Geometry check sheet. Reference: the model listing, model coordinates, mm. Face numbers are marked on the shaded views. A direction names the side the tool comes from. Coordinates: 2 decimals unless noted, no trailing zeros. Order: outer loops, then holes, each group sorted by start corner. A loop starts at its lowest first (then second) coordinate and runs counter-clockwise, first axis right, second up. Notation, with made-up numbers: M 25.5,5 L 61.5,5 A37 cw 61.5,44 Z; hole C 11,-30.5 d3. An arc over 180 degrees is marked long. Use CSV: the item, a comma, the result in double quotes. Start each with the question number.
```python
from build123d import *

# Parameters (mm, degrees)
FURO_ROSCADO_DE_1_4_18_NPSM1_REACH  = 69.594
FURO_ROSCADO_DE_1_4_18_NPSM1_BORE_R = 5.9436
FURO_ROSCADO_DE_1_4_18_NPSM2_REACH  = 82.554
FURO_ROSCADO_DE_1_4_18_NPSM2_BORE_R = 5.9436
ESBO_O4_R                           = 10
CORTE_EXTRUS_O1_DEPTH               = 2
ESBO_O6_R                           = 10
CORTE_EXTRUS_O2_DEPTH               = 2
CORTE_EXTRUS_O3_DEPTH               = 79.42193586


with BuildPart() as part:
    # Esboço1 → Revolução1 (revolve)
    with BuildSketch(Plane.XY, mode=Mode.PRIVATE) as revolu_o1_sk:
        Polygon((9, 32), (25, 32), (25, -38), (0, -38), (0, -34), (9, -34), align=None)
    revolve(revolu_o1_sk.sketch.rotate(Axis((0, 0, 0), (0, 1, 0)), 90), axis=Axis((0, 0, 0), (0, 1, 0)))

    # Furo roscado de 1/4-18 NPSM1 bore (on position points) → Furo roscado de 1/4-18 NPSM1 (cut, up to next)
    with BuildSketch(Plane(origin=(-25, 0, 0), x_dir=(0, 0, -1), z_dir=(-1, 0, 0)), mode=Mode.PRIVATE) as furo_roscado_de_1_4_18_npsm1_sk1:
        Circle(FURO_ROSCADO_DE_1_4_18_NPSM1_BORE_R)
    furo_roscado_de_1_4_18_npsm1_tool1 = extrude(furo_roscado_de_1_4_18_npsm1_sk1.sketch, amount=-FURO_ROSCADO_DE_1_4_18_NPSM1_REACH, mode=Mode.PRIVATE) & part.part
    add(furo_roscado_de_1_4_18_npsm1_tool1.solids().sort_by_distance((-25, 0, 0))[0], mode=Mode.SUBTRACT)

    # Furo roscado de 1/4-18 NPSM2 bore (on position points) → Furo roscado de 1/4-18 NPSM2 (cut, up to next)
    with BuildSketch(Plane(origin=(25, 20, 0), x_dir=(0, 0, 1), z_dir=(1, 0, 0)), mode=Mode.PRIVATE) as furo_roscado_de_1_4_18_npsm2_sk1:
        Circle(FURO_ROSCADO_DE_1_4_18_NPSM2_BORE_R)
    furo_roscado_de_1_4_18_npsm2_tool1 = extrude(furo_roscado_de_1_4_18_npsm2_sk1.sketch, amount=-FURO_ROSCADO_DE_1_4_18_NPSM2_REACH, mode=Mode.PRIVATE) & part.part
    # Furo roscado de 1/4-18 NPSM2 bore (on position points) → Furo roscado de 1/4-18 NPSM2 (cut, up to next)
    with BuildSketch(Plane(origin=(25, 20, 0), x_dir=(0, 0, 1), z_dir=(1, 0, 0)), mode=Mode.PRIVATE) as furo_roscado_de_1_4_18_npsm2_sk2:
        with Locations((0, 40)):
            Circle(FURO_ROSCADO_DE_1_4_18_NPSM2_BORE_R)
    furo_roscado_de_1_4_18_npsm2_tool2 = extrude(furo_roscado_de_1_4_18_npsm2_sk2.sketch, amount=-FURO_ROSCADO_DE_1_4_18_NPSM2_REACH, mode=Mode.PRIVATE) & part.part
    add(furo_roscado_de_1_4_18_npsm2_tool1.solids().sort_by_distance((25, 20, 0))[0], mode=Mode.SUBTRACT)
    add(furo_roscado_de_1_4_18_npsm2_tool2.solids().sort_by_distance((25, -20, 0))[0], mode=Mode.SUBTRACT)

    # Esboço4 → Corte-extrusão1 (cut)
    with BuildSketch(Plane(origin=(-25, 0, 0), x_dir=(0, 0, -1), z_dir=(1, 0, 0))):
        Circle(ESBO_O4_R)
    extrude(amount=CORTE_EXTRUS_O1_DEPTH, mode=Mode.SUBTRACT)

    # Esboço6 → Corte-extrusão2 (cut)
    with BuildSketch(Plane(origin=(25, 0, 0), x_dir=(0, 0, -1), z_dir=(1, 0, 0))):
        with Locations((0, 20)):
            Circle(ESBO_O6_R)
        with Locations((0, -20)):
            Circle(ESBO_O6_R)
    extrude(amount=-CORTE_EXTRUS_O2_DEPTH, mode=Mode.SUBTRACT)

    # Esboço7 → Corte-extrusão3 (cut, through all)
    with BuildSketch(Plane(origin=(0, 32, 0), x_dir=(1, 0, 0), z_dir=(0, 1, 0))):
        with BuildLine():
            Line((-20.712315177, 14), (20.712315177, 14))
            ThreePointArc((20.712315177, 14), (0, 25), (-20.712315177, 14))
        make_face()
        with BuildLine():
            Line((-20.712315177, -14), (20.712315177, -14))
            ThreePointArc((20.712315177, -14), (0, -25), (-20.712315177, -14))
        make_face()
    extrude(amount=-CORTE_EXTRUS_O3_DEPTH, mode=Mode.SUBTRACT)


solid = part.part
```
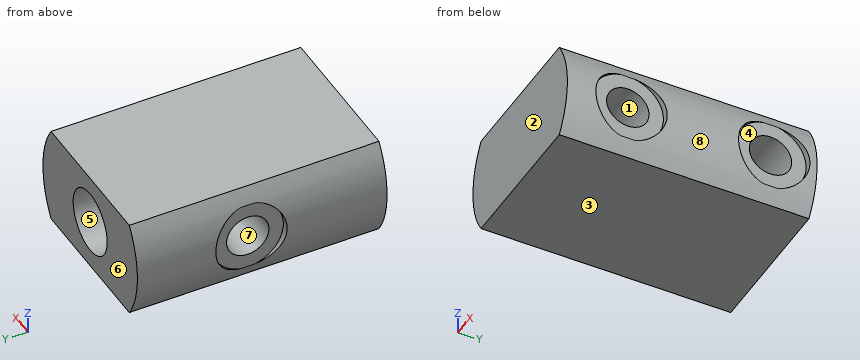
1) Gauge pin test, flat ends, axial feed: P1, Ø7, axis at y = 0, z = 0, coming from the -X side; P2, Ø6, axis at y = -21.5, z = -7.5, coming from the -X side; P3, Ø12, axis at y = 10.5, z = -6.5, coming from the -X side (3 decimals). Record the tip position at first contact, or that the pin passes through.
2) Set-up check for the marked faces 4, 5, 6, 7 and 8: record each of +Z, -Z, +X, -X, +Y, -Y from which the full face is reachable in a straight line by a thin tool's end or side.
3) Draft check along Y on the marked faces 1, 2 and 3. Enter one of: +Y half, -Y half, draft (parallel to the pull), parting line (faces both ways), or undercut.
4) Section check A-A on z = 0. State how many separate pieces and enclosed holes the cut face has, then the cut area to 3 significant figures.
5) Section check B-B on y = 0. Record the boundary of the cut face in (x, z), then the cut area to 3 significant figures.
6) Section check C-C on x = 0. Record the boundary of the cut face in (y, z).
7) Section check D-D on y = -8.5. Record the boundary of the cut face in (x, z), then the cut area to 3 significant figures.
8) Material ranges on line 1 along Y through (x, z) = (18, 0); line 2 along X through (y, z) = (-7.5, -0.25); line 3 along X through (y, z) = (-12.5, 0), recorded low to high.
Results are:
1,P1,"stops at x = 8.29"
1,P2,"stops at x = -24.59"
1,P3,"stops at x = -24.995"
2,face 4,"+X"
2,face 5,"+Y"
2,face 6,"+Z, -Z, +X, -X, +Y"
2,face 7,"-X"
2,face 8,"+X, +Y, -Y"
3,face 1,"undercut"
3,face 2,"-Y half"
3,face 3,"draft"
4,separate pieces,"4"
4,enclosed holes,"0"
4,area,"1,690 mm²"
5,outline,"M -23,-9.8 A25 ccw -20.71,-14 L 20.71,-14 A25 ccw 20.71,14 L -20.71,14 A25 ccw -23,9.8 L -23,5.94 L -6.76,5.94 A9 cw long -6.76,-5.94 L -23,-5.94 Z"
5,area,"867 mm²"
6,outline,"M -38,-14 L 32,-14 L 32,-9 L -34,-9 L -34,9 L 32,9 L 32,14 L -38,14 Z"
7,outline,"M -24.44,-5.27 A25 ccw -20.71,-14 L 20.71,-14 A25 ccw 20.71,14 L -20.71,14 A25 ccw -24.44,5.27 L -23,5.27 L -23,-5.27 Z; hole C 0,0 d18"
7,area,"1,050 mm²"
8,line 1,"y = -38 to -25.94, -14.06 to 14.06, 25.94 to 32"
8,line 2,"x = -23 to -9, 9 to 25"
8,line 3,"x = -25 to -9, 9 to 23"
